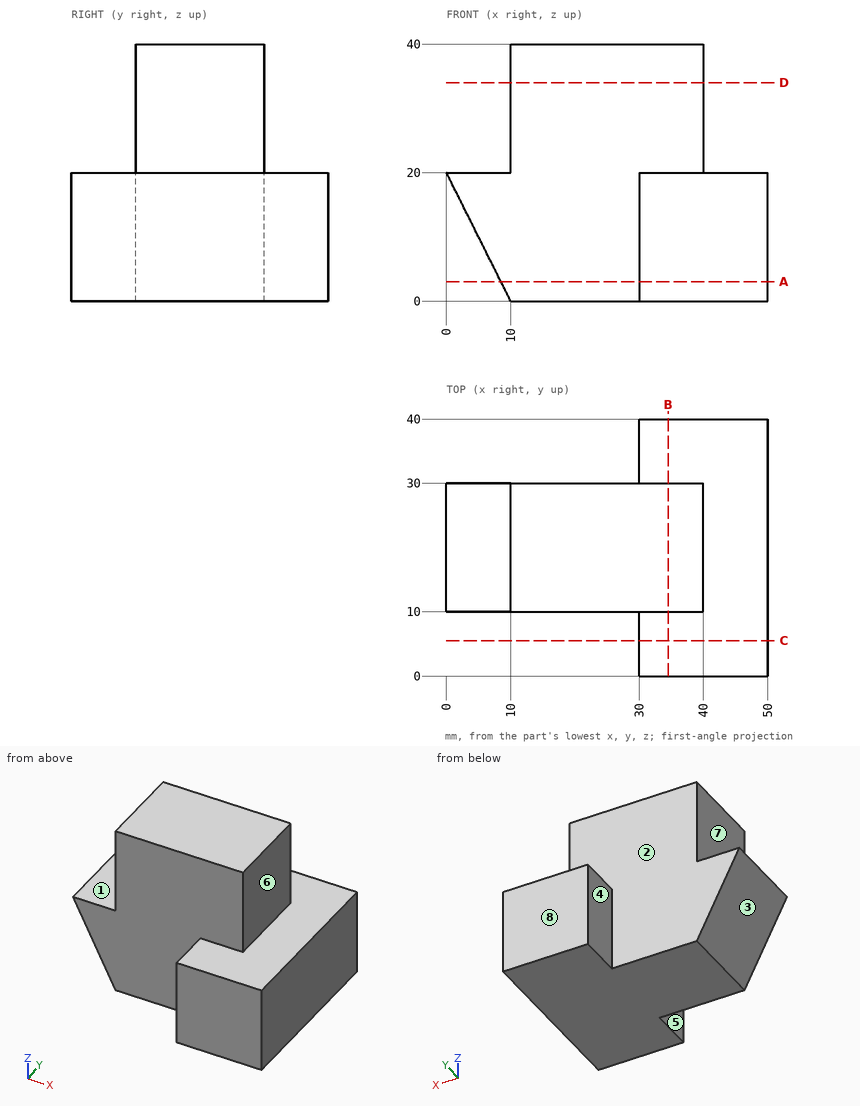
Input: dimensioned drawing with shaded views. Units: mm. Origin: part minimum x, y, z. A direction names the side the tool comes from. Round coordinates to 2 decimals unless told otherwise and drop trailing zeros. Order: outer loops, then holes, each group sorted by start corner. A loop starts at its lowest first (then second) coordinate and runs counter-clockwise, first axis right, second up. Notation, with made-up numbers: (-34.5, -37) - (23.5, -37) arc R15 cw to (23.5, -11) - close; hole circle Ø3 at (38, -24.5). An arc over 180 degrees is marked (long way). Write item = value, one per line. Start each with the question number.
Q1. Cut plane B-B on x = 34.5. Return the cut outline in (y, z), and give its area (3 significant figures).
Q2. Cut plane A-A on z = 3. Return the cut outline in (x, y), and give its area (3 significant figures).
Q3. Access query for the marked faces 4, 5, 6, 7 and 8. Directions: +Z, -Z, +X, -X, +Y, -Y. A direction counts if a zero-diameter tool reaches every point of the face in a straight line with its end or side. Return the directions, or none.
Q4. Ray query, line 1 (Y direction, x = 15, z = 13); line 2 (X direction, y = 36, z = 3.5); line 3 (Z direction, x = 34, y = 4). Return the intervals inside material, ascending. Write a range as from..to.
Q5. Cut plane D-D on z = 34. Return the cut outline in (x, y).
Q6. Pin query (flat end, axial travel): pin 1 (10 mm diameter, centred on x = 15, z = 28, fed in from -Y); pin 2 (8 mm diameter, centred on y = 33, z = 13, fed in from -X); pin 3 (22 mm diameter, centred on y = 19, z = 33, fed in from +X). Return the tip coordinate at first contact, or that it passes through.
Q7. Cut plane C-C on y = 5.5. Return the cut outline in (x, z), and give its area (3 significant figures).
Q8. Pull-direction query (Z, two-part tool) for the marked faces 1, 2 and 3; classes: +Z half, -Z half, draft (parallel to the pull), parting line (faces both ways), or undercut.
Outcome:
q1.outline = (0, 0) - (40, 0) - (40, 20) - (30, 20) - (30, 40) - (10, 40) - (10, 20) - (0, 20) - close
q1.area = 1,200 mm^2
q2.outline = (8.5, 10) - (30, 10) - (30, 0) - (50, 0) - (50, 40) - (30, 40) - (30, 30) - (8.5, 30) - close
q2.area = 1,230 mm^2
q3.face_4 = +Z, -Z, -X, +Y
q3.face_5 = +Z, -Z, -X, -Y
q3.face_6 = +Z, +X, +Y, -Y
q3.face_7 = +Z, -X, +Y, -Y
q3.face_8 = +Z, -Z, +X, -X, +Y
q4.line_1 = 10..30
q4.line_2 = 30..50
q4.line_3 = 0..20
q5.outline = (10, 10) - (40, 10) - (40, 30) - (10, 30) - close
q6.pin_1 = 10
q6.pin_2 = 2.18
q6.pin_3 = 40
q7.outline = (30, 0) - (50, 0) - (50, 20) - (30, 20) - close
q7.area = 400 mm^2
q8.face_1 = +Z half
q8.face_2 = draft
q8.face_3 = -Z half
